Geometry: final body of the model. Coordinates: model frame, mm. Face numbers are marked on the shaded views. Give positions to 0.01 mm unless a question says otherwise; leave off trailing zeros. Write each loop counter-clockwise with the first axis right and the second up, starting at its lowest first coordinate (ties: lowest second). Pieces come first, ordered by that corner, then holes. Notation, with made-up numbers: (-13.5, -3.75) -> (15.5, -3.75) arc R29 ccw to (15.5, 16.25) -> close; hole circle Ø5 at (10.25, 77). An arc over 180 degrees is marked (long way). Answer as a JSON object with one key per item and string values.
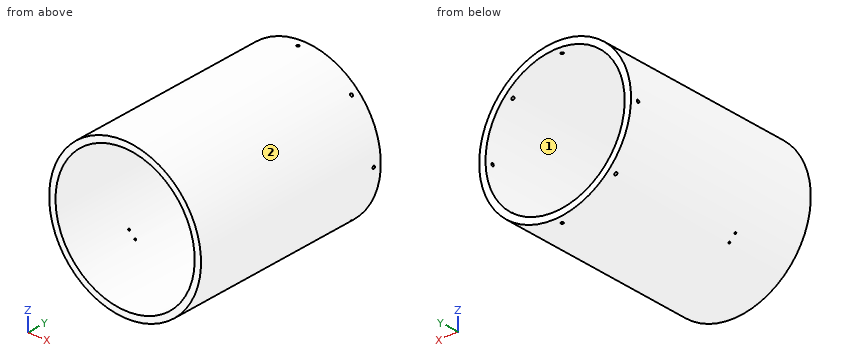
from build123d import *

# Parameters (mm, degrees)
SKETCH1_R                   = 152.4
SKETCH1_R_2                 = 139.7
BOSS_EXTRUDE1_DEPTH         = 406.4
F_10_CLEARANCE_HOLE1_REACH  = 532.368
F_10_CLEARANCE_HOLE1_BORE_R = 2.8067
CIRPATTERN1_COUNT           = 8
F_8_32_TAPPED_HOLE1_REACH   = 550.207
F_8_32_TAPPED_HOLE1_BORE_R  = 1.7272


with BuildPart() as part:
    # Sketch1 → Boss-Extrude1 (new body)
    with BuildSketch(Plane(origin=(0, 0, 0), x_dir=(1, 0, 0), z_dir=(0, 1, 0))):
        with Locations(Location((0, 0, 0), (0, 0, 270))):
            Circle(SKETCH1_R)
        with Locations(Location((0, 0, 0), (0, 0, 270))):
            Circle(SKETCH1_R_2, mode=Mode.SUBTRACT)
    extrude(amount=BOSS_EXTRUDE1_DEPTH)

    # #10 Clearance Hole1 bore → #10 Clearance Hole1 (cut, up to next)
    with BuildSketch(Plane(origin=(152.4, 0, 0), x_dir=(0, 0, -1), z_dir=(1, 0, 0)), mode=Mode.PRIVATE) as f_10_clearance_hole1_sk1:
        with Locations((0, 390.525)):
            Circle(F_10_CLEARANCE_HOLE1_BORE_R)
    f_10_clearance_hole1_tool1 = extrude(f_10_clearance_hole1_sk1.sketch, amount=-F_10_CLEARANCE_HOLE1_REACH, mode=Mode.PRIVATE) & part.part
    f_10_clearance_hole1 = f_10_clearance_hole1_tool1.solids().sort_by_distance((152.4, 390.525, 0))[0]
    add(f_10_clearance_hole1, mode=Mode.SUBTRACT)

    # CirPattern1: #10 Clearance Hole1 ×8 about axis
    cirpattern1_axis = Axis((0, 406.4, 0), (0, 1, 0))
    for i in range(1, CIRPATTERN1_COUNT):
        add(f_10_clearance_hole1.rotate(cirpattern1_axis, i * 360 / CIRPATTERN1_COUNT), mode=Mode.SUBTRACT)

    # #8-32 Tapped Hole1 bore → #8-32 Tapped Hole1 (cut, up to next)
    with BuildSketch(Plane(origin=(-107.763073453, 0, -107.763073453), x_dir=(0, -1, 0), z_dir=(-0.7071067811865464, 0, -0.7071067811865488)), mode=Mode.PRIVATE) as f_8_32_tapped_hole1_sk1:
        with Locations((-127, -8.5725)):
            Circle(F_8_32_TAPPED_HOLE1_BORE_R)
    f_8_32_tapped_hole1_tool1 = extrude(f_8_32_tapped_hole1_sk1.sketch, amount=-F_8_32_TAPPED_HOLE1_REACH, mode=Mode.PRIVATE) & part.part
    # #8-32 Tapped Hole1 bore → #8-32 Tapped Hole1 (cut, up to next)
    with BuildSketch(Plane(origin=(-107.763073453, 0, -107.763073453), x_dir=(0, -1, 0), z_dir=(-0.7071067811865464, 0, -0.7071067811865488)), mode=Mode.PRIVATE) as f_8_32_tapped_hole1_sk2:
        with Locations((-127, 8.5725)):
            Circle(F_8_32_TAPPED_HOLE1_BORE_R)
    f_8_32_tapped_hole1_tool2 = extrude(f_8_32_tapped_hole1_sk2.sketch, amount=-F_8_32_TAPPED_HOLE1_REACH, mode=Mode.PRIVATE) & part.part
    add(f_8_32_tapped_hole1_tool1.solids().sort_by_distance((-101.701401, 127, -113.824746))[0], mode=Mode.SUBTRACT)
    add(f_8_32_tapped_hole1_tool2.solids().sort_by_distance((-113.824746, 127, -101.701401))[0], mode=Mode.SUBTRACT)


solid = part.part
Q1. Cut plane A-A (x = 82). Return the cut outline in (y, z), and give its area (3 significant figures).
Values:
{"outline": "(0, -128.46) -> (406.4, -128.46) -> (406.4, -113.1) -> (0, -113.1) -> close; (0, 113.1) -> (406.4, 113.1) -> (406.4, 128.46) -> (0, 128.46) -> close", "area": "12,500 mm²"}
Q2. Cut plane C-C (y = 55.5). Return the cut outline in (x, z).
Values:
{"outline": "circle Ø304.8 at (0, 0); hole circle Ø279.4 at (0, 0)"}
Q3. Cut plane B-B (z = 71). Return the cut outline in (x, y).
Values:
{"outline": "(-134.85, 0) -> (-120.31, 0) -> (-120.31, 406.4) -> (-134.85, 406.4) -> close; (120.31, 0) -> (134.85, 0) -> (134.85, 406.4) -> (120.31, 406.4) -> close"}
Q4. Mould query, pull axis X, two halves, no side actions, for the marked faces 1 and 2. Classes: pulls with the +X half, pulls with the -X half, needs draft (parallel to the pull), parting line crosses it, or undercut.
Values:
{"face 1": "undercut", "face 2": "parting line crosses it"}
Q5. First-contact query: P1, Ø2, axis at y = 126.5, z = 21, coming from the -X side; P2, Ø6, axis at x = 19, y = 109.5, coming from the -Z side; P3, Ø4, axis at y = 172, z = -9.5, coming from the -X side; P4, Ø4.5, axis at x = 0, y = 390.525, coming from the -Z side. Flat tips, straight axial feed; report the tip coordinate or a pass-through.
Values:
{"P1": "x = -151.08", "P2": "z = -151.56", "P3": "x = -152.22", "P4": "through"}
Q6. Material intervals for L1, parallel to Y at x = 0, z = 149; L2, parallel to X at y = 305, z = 0; L3, parallel to X at y = 70, z = 119.5, sorted ascending. Write a range as from..to.
Values:
{"L1": "0..387.72, 393.33..406.4", "L2": "-152.4..-139.7, 139.7..152.4", "L3": "-94.58..-72.36, 72.36..94.58"}
